from build123d import *

# Parameters (mm, degrees)
SKETCH1_W           = 420
SKETCH1_H           = 100
BOSS_EXTRUDE1_DEPTH = 16
SKETCH2_W           = 420
SKETCH2_H           = 246
BOSS_EXTRUDE2_DEPTH = 16
SKETCH3_W           = 420
SKETCH3_H           = 12
SKETCH3_W_2         = 12
SKETCH3_H_2         = 111
SKETCH3_H_3         = 111.25908774
BOSS_EXTRUDE3_DEPTH = 100
SKETCH4_R           = 7.25
CUT_EXTRUDE3_DEPTH  = 16
SKETCH5_R           = 7.25
CUT_EXTRUDE4_DEPTH  = 26


with BuildPart() as part:
    # Sketch1 → Boss-Extrude1 (new body)
    with BuildSketch(Plane(origin=(0, 0, 0), x_dir=(1, 0, 0), z_dir=(0, 1, 0))):
        with Locations((0, -50)):
            Rectangle(SKETCH1_W, SKETCH1_H)
    extrude(amount=BOSS_EXTRUDE1_DEPTH)

    # Sketch2 → Boss-Extrude2 (add)
    with BuildSketch(Plane.XY):
        with Locations((0, 139)):
            Rectangle(SKETCH2_W, SKETCH2_H)
    extrude(amount=BOSS_EXTRUDE2_DEPTH)

    # Sketch3 → Boss-Extrude3 (add)
    with BuildSketch(Plane.XY):
        with Locations((0, 256)):
            Rectangle(SKETCH3_W, SKETCH3_H)
        with Locations((-204, 194.5)):
            Rectangle(SKETCH3_W_2, SKETCH3_H_2)
        with Locations((-102, 194.5)):
            Rectangle(SKETCH3_W_2, SKETCH3_H_2)
        with Locations((0, 194.5)):
            Rectangle(SKETCH3_W_2, SKETCH3_H_2)
        with Locations((0, 133)):
            Rectangle(SKETCH3_W, SKETCH3_H)
        with Locations((-204, 71.5)):
            Rectangle(SKETCH3_W_2, SKETCH3_H_2)
        with Locations((-102, 71.37045613)):
            Rectangle(SKETCH3_W_2, SKETCH3_H_3)
        with Locations((204, 71.5)):
            Rectangle(SKETCH3_W_2, SKETCH3_H_2)
        with Locations((204, 194.5)):
            Rectangle(SKETCH3_W_2, SKETCH3_H_2)
        with Locations((0, 71.5)):
            Rectangle(SKETCH3_W_2, SKETCH3_H_2)
        with Locations((102, 194.5)):
            Rectangle(SKETCH3_W_2, SKETCH3_H_2)
        with Locations((102, 71.5)):
            Rectangle(SKETCH3_W_2, SKETCH3_H_2)
    extrude(amount=BOSS_EXTRUDE3_DEPTH)

    # Sketch4 → Cut-Extrude3 (cut)
    with BuildSketch(Plane(origin=(0, 0, 0), x_dir=(1, 0, 0), z_dir=(0, 1, 0))):
        with Locations(Location((-153, -75, 0), (0, 0, 270))):
            Circle(SKETCH4_R)
        with Locations(Location((-51, -75, 0), (0, 0, 270))):
            Circle(SKETCH4_R)
        with Locations(Location((51, -75, 0), (0, 0, 270))):
            Circle(SKETCH4_R)
        with Locations(Location((153, -75, 0), (0, 0, 270))):
            Circle(SKETCH4_R)
    extrude(amount=CUT_EXTRUDE3_DEPTH, mode=Mode.SUBTRACT)

    # Sketch5 → Cut-Extrude4 (cut)
    with BuildSketch(Plane.ZY.offset(-198)):
        with Locations((80, 212)):
            Circle(SKETCH5_R)
        with Locations((80, 162)):
            Circle(SKETCH5_R)
        with Locations((80, 100)):
            Circle(SKETCH5_R)
        with Locations((80, 50)):
            Circle(SKETCH5_R)
    cut_extrude4 = extrude(amount=-CUT_EXTRUDE4_DEPTH, mode=Mode.SUBTRACT)

    # Mirror1: Cut-Extrude4 across plane
    add(cut_extrude4.mirror(Plane(origin=(0, 0, 0), x_dir=(0, 0, 1), z_dir=(1, 0, 0))), mode=Mode.SUBTRACT)


solid = part.part
The model under review builds one solid part; all positions refer to its coordinate system, in mm. A direction names the side the tool comes from. Round coordinates to 2 decimals unless told otherwise and drop trailing zeros. Write each loop counter-clockwise with the first axis right and the second up, starting at its lowest first coordinate (ties: lowest second). Pieces come first, ordered by that corner, then holes. Notation, with made-up numbers: M 85,2.5 L 91,2.5 A13 cw 91,18.5 Z; hole C 69,28.5 d10. An arc over 180 degrees is marked long. Answer as CSV lines item,"result". Start each with the question number.
Q1. Consider section C-C, the plane y = 113. Give the boundary of the cut face in (x, z).
Q2. Consider section B-B, the plane y = 212. Give the boundary of the cut face in (x, z).
Q3. Wall thickness on line 1 along Y through (x, z) = (-11, 19.5); line 2 along X through (y, z) = (5, 75); line 3 along Y through (x, z) = (206.5, 80): over which ranges is each line inside the solid? List them lowest first.
Q4. Tool access review of faces 1 (the face through (-203.916, 45.588, 74.247)), 2 (the face through (-52, 127, 57)), 3 (the face through (203.916, 166.9, 74.656)): name each direction out of +Z, -Z, +X, -X, +Y, -Y from which nothing blocks a thin tool from reaching the whole face with its end or side.
Q5. The part is to be moulded in two halves that separate along Z. For faces 4 (the face through (-203.916, 216.9, 74.656)), 5 (the face through (-3, 133, 0)), 6 (the face through (-96, 71, 57)), say which applies: +Z half, -Z half, draft (parallel to the pull), parting line (faces both ways), or undercut.
Q6. Consider section A-A, the plane x = 153. Give the boundary of the cut face in (y, z), then the cut area to 3 significant figures.
Q7. Clearance check with a flat-ended pin moving along its axis: P1, Ø1, axis at x = 153.5, y = 88, coming from the +Z side. State where the tip first meets the part, or that it passes through.
Q8. Consider section D-D, the plane z = 61.5. State how many separate pieces and enclosed holes the cut face has, then the cut area to 3 significant figures.
Result set:
1,outline,"M -210,0 L 210,0 L 210,100 L 198,100 L 198,16 L 108,16 L 108,100 L 96,100 L 96,16 L 6,16 L 6,100 L -6,100 L -6,16 L -96,16 L -96,100 L -108,100 L -108,16 L -198,16 L -198,100 L -210,100 Z"
2,outline,"M -210,0 L 210,0 L 210,72.75 L 198,72.75 L 198,16 L 108,16 L 108,100 L 96,100 L 96,16 L 6,16 L 6,100 L -6,100 L -6,16 L -96,16 L -96,100 L -108,100 L -108,16 L -198,16 L -198,72.75 L -210,72.75 Z; M -210,87.25 L -198,87.25 L -198,100 L -210,100 Z; M 198,87.25 L 210,87.25 L 210,100 L 198,100 Z"
3,line 1,"y = 0 to 16, 127 to 139, 250 to 262"
3,line 2,"x = -210 to -160.25, -145.75 to -58.25, -43.75 to 43.75, 58.25 to 145.75, 160.25 to 210"
3,line 3,"y = 0 to 42.75, 57.25 to 92.75, 107.25 to 154.75, 169.25 to 204.75, 219.25 to 262"
4,face 1,"-X"
4,face 2,"+Z"
4,face 3,"+X"
5,face 4,"undercut"
5,face 5,"-Z half"
5,face 6,"draft"
6,outline,"M 0,0 L 262,0 L 262,100 L 250,100 L 250,16 L 139,16 L 139,100 L 127,100 L 127,16 L 16,16 L 16,67.75 L 0,67.75 Z; M 0,82.25 L 16,82.25 L 16,100 L 0,100 Z"
6,area,"7,320 mm²"
7,P1,"stops at z = 16"
8,separate pieces,"1"
8,enclosed holes,"8"
8,area,"30,100 mm²"
